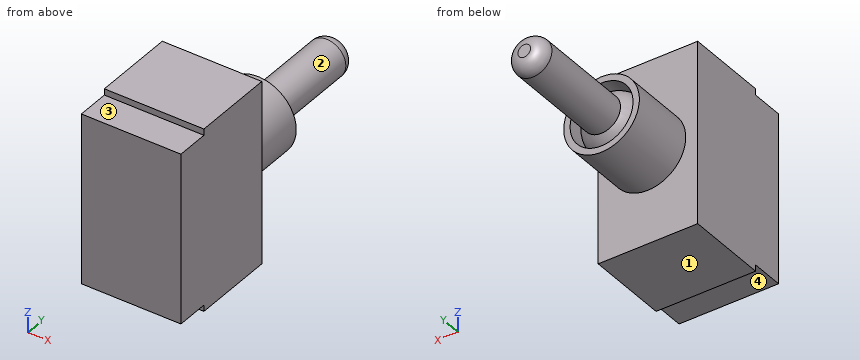
```python
from build123d import *

# Parameters (mm, degrees)
SKETCH1_W           = 15.8
SKETCH1_H           = 29
BOSS_EXTRUDE1_DEPTH = 13.1
SKETCH2_R           = 6
BOSS_EXTRUDE2_DEPTH = 10.5
SKETCH4_R           = 5
CUT_EXTRUDE1_DEPTH  = 4
SKETCH5_R           = 3
BOSS_EXTRUDE3_DEPTH = 21.5
REVOLVE2_ANGLE      = 180
FILLET1_R           = 2
SKETCH6_W           = 15.8
SKETCH6_H           = 27
BOSS_EXTRUDE4_DEPTH = 5.2


with BuildPart() as part:
    # Sketch1 → Boss-Extrude1 (new body)
    with BuildSketch(Plane(origin=(0, 0, 0), x_dir=(1, 0, 0), z_dir=(0, 1, 0))):
        Rectangle(SKETCH1_W, SKETCH1_H)
    extrude(amount=BOSS_EXTRUDE1_DEPTH)

    # Sketch2 → Boss-Extrude2 (add)
    with BuildSketch(Plane(origin=(0, 13.1, 0), x_dir=(1, 0, 0), z_dir=(0, 1, 0))):
        Circle(SKETCH2_R)
    extrude(amount=BOSS_EXTRUDE2_DEPTH)

    # Sketch4 → Cut-Extrude1 (cut)
    with BuildSketch(Plane(origin=(0, 23.6, 0), x_dir=(1, 0, 0), z_dir=(0, 1, 0))):
        Circle(SKETCH4_R)
    extrude(amount=-CUT_EXTRUDE1_DEPTH, mode=Mode.SUBTRACT)

    # Sketch5 → Boss-Extrude3 (add)
    with BuildSketch(Plane(origin=(0, 19.6, 0), x_dir=(1, 0, 0), z_dir=(0, 1, 0))):
        Circle(SKETCH5_R)
    extrude(amount=BOSS_EXTRUDE3_DEPTH)

    # Sketch3 → Revolve2 (revolve)
    with BuildSketch(Plane(origin=(0, 19.6, 0), x_dir=(1, 0, 0), z_dir=(0, 1, 0))):
        with BuildLine():
            Line((0, -5), (0, 5))
            ThreePointArc((0, 5), (-5, 0), (0, -5))
        make_face()
    revolve(axis=Axis((0, 19.6, 6), (0, 0, -1)), revolution_arc=REVOLVE2_ANGLE)

    # Fillet1
    fillet1_edges = [part.edges().sort_by_distance(p)[0] for p in [
        (-3, 41.1, 0),
    ]]
    fillet(fillet1_edges, radius=FILLET1_R)

    # Sketch6 → Boss-Extrude4 (add)
    with BuildSketch(Plane.XZ):
        Rectangle(SKETCH6_W, SKETCH6_H)
    extrude(amount=BOSS_EXTRUDE4_DEPTH)


solid = part.part
```
The model under review builds one solid part; all positions refer to its coordinate system, in mm. Face numbers are marked on the shaded views. A direction names the side the tool comes from. Coordinates: 2 decimals unless noted, no trailing zeros. Write each loop counter-clockwise with the first axis right and the second up, starting at its lowest first coordinate (ties: lowest second). Pieces come first, ordered by that corner, then holes. Notation, with made-up numbers: (43.5, 82) -> (63.5, 82) arc R28 ccw to (63.5, 103) -> close; hole circle Ø8 at (-11, 47.25). An arc over 180 degrees is marked (long way). One line per item, written item: value. Start each with the question number.
Q1. Add section C-C, the plane x = -3.5. Give the boundary of the cut face in (y, z).
Q2. For the marked faces 1, 2, 3 and 4, list the 3-axis set-ups (+Z, -Z, +X, -X, +Y, -Y) from which the entire face can be reached by the end or side of a thin tool; tool diameter is ignored.
Q3. Add section B-B, the plane y = 14.5. Give the boundary of the cut face in (x, z).
Q4. Add section A-A, the plane x = -6.5. Give the boundary of the cut face in (y, z), then the cut area to 3 significant figures.
Q5. Add section D-D, the plane y = 27.5. Give the boundary of the cut face in (x, z), then the cut area to 3 significant figures.
Q6. Clearance check with flat-ended pins moving along their axes: P1, Ø0.5, axis at x = 1, z = 14, coming from the -Y side; P2, Ø3.5, axis at x = -2.5, z = 2, coming from the +Y side; P3, Ø2.5, axis at x = -4, y = -2, coming from the -Z side. State where each tip first meets the part, or that it passes through.
Q7. To check wall thickness, follow probe 1 along X at (y, z) = (21.6, 0); probe 2 along Z at (x, y) = (0, 22.7); probe 3 along Y at (x, z) = (-4.5, 6.5). State the ranges of each line that lie inside material, in increasing order.
Response:
1. outline: (-5.2, -13.5) -> (0, -13.5) -> (0, -14.5) -> (13.1, -14.5) -> (13.1, -4.87) -> (23.6, -4.87) -> (23.6, -3.57) -> (19.6, -3.57) arc R3.57 ccw to (19.6, 3.57) -> (23.6, 3.57) -> (23.6, 4.87) -> (13.1, 4.87) -> (13.1, 14.5) -> (0, 14.5) -> (0, 13.5) -> (-5.2, 13.5) -> close
2. face 1: -Z, +X, -X, +Y, -Y
2. face 2: +Y
2. face 3: +Z, +X, -X, -Y
2. face 4: -Z, +X, -X, -Y
3. outline: circle Ø12 at (0, 0)
4. outline: (-5.2, -13.5) -> (0, -13.5) -> (0, -14.5) -> (13.1, -14.5) -> (13.1, 14.5) -> (0, 14.5) -> (0, 13.5) -> (-5.2, 13.5) -> close
4. area: 520 mm²
5. outline: circle Ø6 at (0, 0)
5. area: 28.3 mm²
6. P1: y = 0
6. P2: y = 41.05
6. P3: z = -13.5
7. probe 1: -6 to -5, -4.58 to 4.58, 5 to 6
7. probe 2: -6 to -5, -3.92 to 3.92, 5 to 6
7. probe 3: -5.2 to 13.1
